Design review of the part shown in the three views and the two pictorial views. Dimensions are in mm from the part's minimum x, y and z. A direction names the side the tool comes from. Coordinates: 2 decimals unless noted, no trailing zeros. Loops run counter-clockwise (first coordinate to the right, second up) from the corner with the lowest first, then second, coordinate; pieces in that order, holes last. Notation, with made-up numbers: M 21.25,-9.5 L 67.25,-9.5 A20 ccw 67.25,-4.5 Z; hole C 44,23 d5. An arc over 180 degrees is marked long. Write item = value, one per line. Start each with the question number.
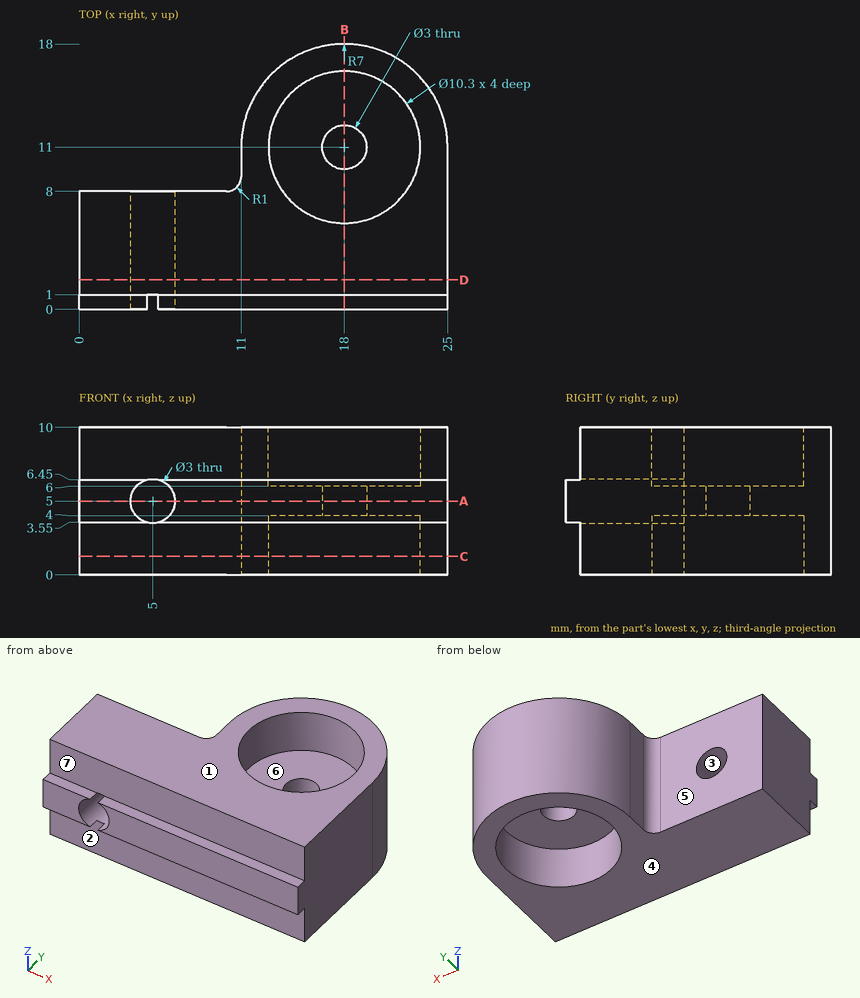
(1) Take a section at C-C (z = 1.25). State the section outline as (x, y) points, plus the area to 3 significant figures.
(2) Tool access review of the marked faces 5, 6 and 7: name each direction out of +Z, -Z, +X, -X, +Y, -Y from which nothing blocks a thin tool from reaching the whole face with its end or side.
(3) Take a section at A-A (z = 5). State the section outline as (x, y) points, plus the area to 3 significant figures.
(4) Take a section at D-D (y = 2). State the section outline as (x, z) points, plus the area to 3 significant figures.
(5) Insertion check: pin 1 (3.5 mm diameter, centred on x = 5, z = 5, fed in from +Y); pin 2 (0.5 mm diameter, centred on x = 15, y = 0.5, fed in from -Z); pin 3 (2 mm diameter, centred on x = 11.5, y = 16, fed in from -Z) (1 decimal); pin 4 (9.5 mm diameter, centred on x = 18, y = 11, fed in from -Z). Each pin has a flat end and moves straight along its axis. Give the tip position at first contact, or say it passes through.
(6) To check wall thickness, follow L1, parallel to Y at x = 18, z = 3.1; L2, parallel to X at y = 11, z = 5.25; L3, parallel to Y at x = 18, z = 5.5. State the ranges of each line that lie inside material, in increasing order.
(7) Mouldability with a two-part tool opening along Z and no side actions: class the marked faces 1, 2, 3 and 4 as +Z half, -Z half, draft (parallel to the pull), parting line (faces both ways), or undercut.
(8) Take a section at B-B (x = 18). State the section outline as (y, z) points, plus the area to 3 significant figures.
Results list:
q1.outline = M 0,1 L 25,1 L 25,11 A7 ccw 11,11 L 11,9 A1 cw 10,8 L 0,8 Z; hole C 18,11 d10.3
q1.area = 211 mm^2
q2.face_5 = +Z, -Z, -X, +Y
q2.face_6 = +Z
q2.face_7 = +Z, +X, -X, -Y
q3.outline = M 0,0 L 3.5,0 L 3.5,8 L 0,8 Z; M 6.5,0 L 25,0 L 25,11 A7 ccw 11,11 L 11,9 A1 cw 10,8 L 6.5,8 Z; hole C 18,11 d3
q3.area = 288 mm^2
q4.outline = M 0,0 L 25,0 L 25,10 L 0,10 Z; hole C 5,5 d3
q4.area = 243 mm^2
q5.pin_1 = 8
q5.pin_2 = 3.55
q5.pin_3 = through
q5.pin_4 = 4
q6.L1 = 1 to 5.85, 16.15 to 18
q6.L2 = 11 to 16.5, 19.5 to 25
q6.L3 = 0 to 9.5, 12.5 to 18
q7.face_1 = +Z half
q7.face_2 = draft
q7.face_3 = undercut
q7.face_4 = -Z half
q8.outline = M 0,3.55 L 1,3.55 L 1,0 L 5.85,0 L 5.85,4 L 9.5,4 L 9.5,6 L 5.85,6 L 5.85,10 L 1,10 L 1,6.45 L 0,6.45 Z; M 12.5,4 L 16.15,4 L 16.15,0 L 18,0 L 18,10 L 16.15,10 L 16.15,6 L 12.5,6 Z
q8.area = 84.5 mm^2
